Drawing for the job (mm, zero at the part's lowest x, y, z). A direction names the side the tool comes from. Coordinates: 2 decimals unless noted, no trailing zeros. Loops run counter-clockwise (first coordinate to the right, second up) from the corner with the lowest first, then second, coordinate; pieces in that order, holes last. Notation, with made-up numbers: (63, -34) -> (110, -34) arc R23 cw to (110, 3) -> close; hole circle Ø2 at (0.25, 78.5). An arc over 180 degrees is marked (long way). Write each question's results on one line, items separated by ' | '.
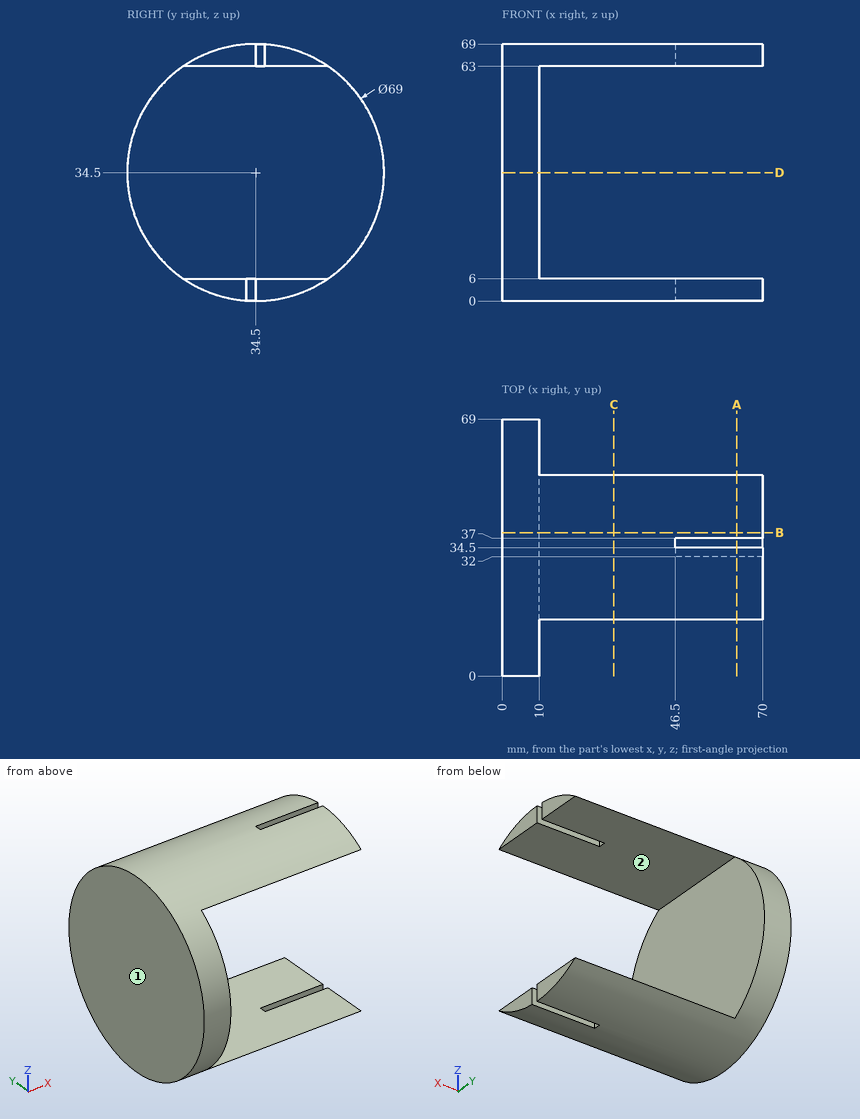
1) Drill centre lines: L1, parallel to Z at x = 19, y = 34; L2, parallel to Z at x = 50, y = 25; L3, parallel to X at y = 47, z = 25. Where is each one in solid material? Low to high. Write a range as from..to.
Outcome:
L1: z = 0..6, 63..69 | L2: z = 1.33..6, 63..67.67 | L3: x = 0..10
2) Which spindle directions (+Z, -Z, +X, -X, +Y, -Y) get a long thin tool onto all of the face, cutting with end or side? Do the marked faces 1 and 2. Say none if no direction does.
Outcome:
face 1: +Z, -Z, -X, +Y, -Y | face 2: +X, +Y, -Y
3) Slice it at B-B (y = 38.5). Write the cut outline in (x, z).
Outcome:
outline: (0, 0.23) -> (70, 0.23) -> (70, 6) -> (10, 6) -> (10, 63) -> (70, 63) -> (70, 68.77) -> (0, 68.77) -> close
4) Slice it at A-A (x = 63). Write the cut outline in (y, z), then the cut area to 3 significant figures.
Outcome:
outline: (15.06, 6) arc R34.5 ccw to (32, 0.09) -> (32, 6) -> close; (15.06, 63) -> (34.5, 63) -> (34.5, 69) arc R34.5 ccw to start; (34.5, 0) arc R34.5 ccw to (53.94, 6) -> (34.5, 6) -> close; (37, 63) -> (53.94, 63) arc R34.5 ccw to (37, 68.91) -> close | area: 287 mm^2
5) Slice it at D-D (z = 34.5). Write the cut outline in (x, y), then the cut area to 3 significant figures.
Outcome:
outline: (0, 0) -> (10, 0) -> (10, 69) -> (0, 69) -> close | area: 690 mm^2
6) Slice it at C-C (x = 30). Write the cut outline in (y, z).
Outcome:
outline: (15.06, 6) arc R34.5 ccw to (53.94, 6) -> close; (15.06, 63) -> (53.94, 63) arc R34.5 ccw to start
7) Pin check, flat tips, straight feed: pin 1 (5 mm diameter, centred on x = 39, y = 11, fed in from -Z); pin 2 (6 mm diameter, centred on x = 43, z = 61.5, fed in from +Y); pin 3 (4 mm diameter, centred on x = 29, y = 32, fed in from -Z); pin 4 (0.8 mm diameter, centred on y = 33.5, z = 2.5, fed in from +X). Stop position of each tip, or through.
Outcome:
pin 1: passes through | pin 2: stops at y = 53.94 | pin 3: stops at z = 0 | pin 4: stops at x = 46.5
